Work out the finished part from the listing and answer in its coordinate system (mm). A direction names the side the tool comes from. Give positions to 0.01 mm unless a question says otherwise; leave off trailing zeros. Loops run counter-clockwise (first coordinate to the right, second up) from the corner with the lowest first, then second, coordinate; pieces in that order, holes last. Notation, with made-up numbers: M 79.5,26 L 123.5,26 A20 ccw 123.5,51 Z; hole C 43,-37.75 d9. An arc over 180 degrees is marked long. Write item = value, one per line. Start each with the question number.
1. Section D-D on z = 9 is taken. Determine the outline of the cut face in (x, y).
2. Section B-B on x = -122.25 is taken. Determine the outline of the cut face in (y, z).
3. Consider L1, parallel to Y at x = -117.6, z = 3.25; L2, parallel to Y at x = -117.6, z = 4; L3, parallel to Y at x = -119, z = 5.75. Determine where each line is inside the solid, lowest interval first. Write a range as [from, to].
4. The mould has two halves that part along X. Classify faces 3 (the face through (-110.75, 14.53, 5.31)), 4 (the face through (-118, 15.6, 2)), 5 (the face through (-120, -13, 8)), 6 (the face through (-128.8, 7.1, 7.4)): released by +X, released by -X, zero draft, split by the parting line, or undercut.
5. Section C-C on y = -12.85 is taken. Determine the outline of the cut face in (x, z), plus the area to 3 significant figures.
6. Flat-ended cylindrical pins translate along their axes: pin 1 Ø3 at (x, y) = (-116, -12) entering from +Z; pin 2 Ø6 at (x, y) = (-119, -12.5) entering from -Z; pin 3 Ø6 at (x, y) = (-116, 13.5) entering from +Z; pin 4 Ø4 at (x, y) = (-117.6, -12.85) entering from +Z. Find the tip coordinate at first contact, or state that the pin passes through.
7. For faces 1 (the face through (-117.5, 9.85, 10.31)), 2 (the face through (-115.85, 12.93, 3.94)), determine the directions among +Z, -Z, +X, -X, +Y, -Y from which every point of the face is accessible in a straight line to the end or side of a thin tool.
8. Section A-A on z = 4.5 is taken. Determine the outline of the cut face in (x, y).
```python
from build123d import *

# Parameters (mm, degrees)
BOSS_EXTRUDE1_DEPTH = 15
SKETCH3_R           = 5
CUT_EXTRUDE1_DEPTH  = 30.486936791
SKETCH5_R           = 1.75
CUT_EXTRUDE3_DEPTH  = 131.953306572
CUT_EXTRUDE4_START  = -8
SKETCH6_R           = 3
CUT_EXTRUDE4_DEPTH  = 123.953306572
FILLET1_START       = -130
FILLET1_DEPTH       = 19.4


with BuildPart() as part:
    # Sketch1 → Boss-Extrude1 (new body)
    with BuildSketch(Plane.XY):
        with BuildLine():
            Line((-124.6, 14.6), (-128.493415545, 7.856406461))
            ThreePointArc((-128.493415545, 7.856406461), (-128.793116813, 7.132863596), (-128.895339334, 6.356406461))
            Line((-128.895339334, 6.356406461), (-128.895339334, -9.356406461))
            ThreePointArc((-128.895339334, -9.356406461), (-128.793116813, -10.132863596), (-128.493415545, -10.856406461))
            Line((-128.493415545, -10.856406461), (-124.6, -17.6))
            Line((-124.6, -17.6), (-110.6, -17.6))
            Line((-110.6, -17.6), (-110.6, -5))
            Line((-110.6, -5), (-110.6, 5))
            Line((-110.6, 5), (-110.6, 13.771572875))
            ThreePointArc((-110.6, 13.771572875), (-110.752240935, 14.53693974), (-111.185786438, 15.185786438))
            Line((-111.185786438, 15.185786438), (-111.6, 15.6))
            Line((-111.6, 15.6), (-123.6, 15.6))
            Line((-123.6, 15.6), (-124.6, 14.6))
        make_face()
    extrude(amount=BOSS_EXTRUDE1_DEPTH)

    # Sketch3 → Cut-Extrude1 (cut, through all)
    with BuildSketch(Plane(origin=(-110.6, 0, 0), x_dir=(0, 0, -1), z_dir=(1, 0, 0))):
        Circle(SKETCH3_R)
    extrude(amount=-CUT_EXTRUDE1_DEPTH, mode=Mode.SUBTRACT)

    # Sketch5 → Cut-Extrude3 (cut, through all)
    with BuildSketch(Plane(origin=(0, 0, 0), x_dir=(-1, 0, 0), z_dir=(0, 0, -1))):
        with Locations((117.6, 12.85)):
            Circle(SKETCH5_R)
        with Locations((117.6, -12.85)):
            Circle(SKETCH5_R)
    extrude(amount=-CUT_EXTRUDE3_DEPTH, mode=Mode.SUBTRACT)

    # Sketch6 → Cut-Extrude4 (cut, through all)
    with BuildSketch(Plane(origin=(0, 0, 0), x_dir=(-1, 0, 0), z_dir=(0, 0, -1)).offset(CUT_EXTRUDE4_START)):
        with Locations((117.6, 12.85)):
            Circle(SKETCH6_R)
        with Locations((117.6, -12.85)):
            Circle(SKETCH6_R)
    extrude(amount=-CUT_EXTRUDE4_DEPTH, mode=Mode.SUBTRACT)

    # Fillet1: read off the stored shape, not the designer's step
    # Fillet1 outline → Fillet1 (cut)
    with BuildSketch(Plane.YZ.offset(FILLET1_START)):
        with BuildLine():
            ThreePointArc((-17.6, 5), (-14.671067812, 12.071067812), (-7.6, 15))
            Line((-7.6, 15), (-17.6, 15))
            Line((-17.6, 15), (-17.6, 5))
        make_face()
        with BuildLine():
            ThreePointArc((5.6, 15), (12.671067812, 12.071067812), (15.6, 5))
            Line((15.6, 5), (15.6, 15))
            Line((15.6, 15), (5.6, 15))
        make_face()
    extrude(amount=FILLET1_DEPTH, mode=Mode.SUBTRACT)


solid = part.part
```
Verdict:
q1.outline = M -128.9,-9.36 A3 ccw -128.49,-10.86 L -125.08,-16.77 L -110.6,-16.77 L -110.6,13.77 A2 ccw -110.86,14.77 L -115.29,14.77 A3 cw long -119.91,14.77 L -124.43,14.77 L -124.6,14.6 L -128.49,7.86 A3 ccw -128.9,6.36 Z; hole C -117.6,-12.85 d6
q2.outline = M -17.6,0 L -5,0 A5 cw 5,0 L 15.6,0 L 15.6,5 A10 ccw 5.6,15 L -7.6,15 A10 ccw -17.6,5 Z
q3.L1 = [-17.6, -14.6], [-11.1, -3.8], [3.8, 11.1], [14.6, 15.6]
q3.L2 = [-17.6, -14.6], [-11.1, -3], [3, 11.1], [14.6, 15.6]
q3.L3 = [-17.57, -13.9], [-11.8, 11.8], [13.9, 15.57]
q4.face_3 = released by +X
q4.face_4 = zero draft
q4.face_5 = undercut
q4.face_6 = released by -X
q5.outline = M -127.34,0 L -119.35,0 L -119.35,8 L -120.6,8 L -120.6,13.51 L -127.34,13.51 Z; M -115.85,0 L -110.6,0 L -110.6,13.51 L -114.6,13.51 L -114.6,8 L -115.85,8 Z
q5.area = 165 mm2
q6.pin_1 = 14.56
q6.pin_2 = 0
q6.pin_3 = 13.71
q6.pin_4 = 8
q7.face_1 = +Z
q7.face_2 = +Z, -Z
q8.outline = M -128.9,-9.36 A3 ccw -128.49,-10.86 L -124.6,-17.6 L -110.6,-17.6 L -110.6,-2.18 L -128.9,-2.18 Z; M -128.9,2.18 L -110.6,2.18 L -110.6,13.77 A2 ccw -111.19,15.19 L -111.6,15.6 L -123.6,15.6 L -124.6,14.6 L -128.49,7.86 A3 ccw -128.9,6.36 Z; hole C -117.6,-12.85 d3.5; hole C -117.6,12.85 d3.5
